Geometry: final body of the model. Coordinates: model frame, mm. Face numbers are marked on the shaded views. A direction names the side the tool comes from. Round coordinates to 2 decimals unless told otherwise and drop trailing zeros. Write each loop counter-clockwise with the first axis right and the second up, starting at its lowest first coordinate (ties: lowest second). Pieces come first, ordered by that corner, then holes. Notation, with made-up numbers: (56, 78.5) -> (72, 78.5) arc R22 ccw to (72, 99.5) -> close; hole circle Ø5 at (-13, 15.5). An arc over 180 degrees is marked (long way). Use one line per item in the form item = value. Start each with the question number.
1. Cut plane B-B, the plane y = 1.25. Return the cut outline in (x, z) (3 decimals), plus the area to 3 significant figures.
2. Line query: L1, parallel to X at y = 3, z = 19; L2, parallel to Z at x = 11.25, y = 4.5; L3, parallel to Y at x = -4, z = -19.05. Output: solid intervals per line, ascending.
3. Cut plane D-D, the plane z = 5. Return the cut outline in (x, y), plus the area to 3 significant figures.
4. Draft query along X for the marked faces 1, 2, 3 and 4. Return one class per face: pulls with the +X half, pulls with the -X half, needs draft (parallel to the pull), parting line crosses it, or undercut.
5. Pin query (flat end, axial travel): pin 1 Ø3 at (x, z) = (8, 4) entering from -Y; pin 2 Ø9.5 at (y, z) = (-13.5, 3.5) entering from +X. Return the tip coordinate at first contact, or that it passes through.
6. Cut plane A-A, the plane z = -19.05. Return the cut outline in (x, y), plus the area to 3 significant figures.
7. Reachability of the marked faces 5 and 6 from +Z, -Z, +X, -X, +Y, -Y: full face, straight path, thin tool, end or side. Return the list, or none.
8. Cut plane C-C, the plane x = 8.75. Return the cut outline in (y, z).
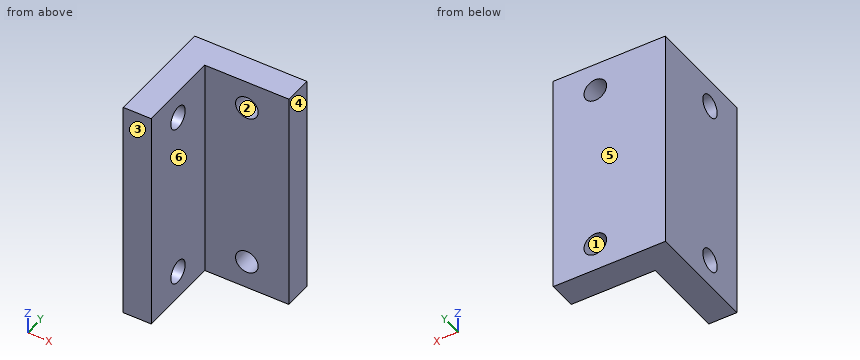
```python
from build123d import *

# Parameters (mm, degrees)
BOSS_EXTRUDE1_DEPTH        = 25.4
F_10_CLEARANCE_HOLE1_D     = 5.1054
F_10_CLEARANCE_HOLE2_D     = 5.1054
F_10_CLEARANCE_HOLE2_DEPTH = 6.35
F_10_CLEARANCE_HOLE2_TIP   = 1.533816902


with BuildPart() as part:
    # Sketch1 → Boss-Extrude1 (new, symmetric)
    with BuildSketch(Plane.XY):
        Polygon((0, 0), (19.05, 0), (19.05, 6.35), (-6.35, 6.35), (-6.35, -19.05), (0, -19.05), align=None)
    extrude(amount=BOSS_EXTRUDE1_DEPTH, both=True)

    # #10 Clearance Hole1 (through all)
    with Locations(Plane(origin=(0, 0, 0), x_dir=(-1, 0, 0), z_dir=(0, -1, 0))):
        with Locations((-9.525, -19.05), (-9.525, 19.05)):
            Hole(F_10_CLEARANCE_HOLE1_D / 2)

    # #10 Clearance Hole2
    with Locations(Plane(origin=(0, 0, 0), x_dir=(0, 0, -1), z_dir=(1, 0, 0))):
        with Locations((19.05, -9.525), (-19.05, -9.525)):
            Hole(F_10_CLEARANCE_HOLE2_D / 2, depth=F_10_CLEARANCE_HOLE2_DEPTH)
            with Locations((0, 0, -(F_10_CLEARANCE_HOLE2_DEPTH + F_10_CLEARANCE_HOLE2_TIP / 2))):  # 118° drill point
                Cone(0, F_10_CLEARANCE_HOLE2_D / 2, F_10_CLEARANCE_HOLE2_TIP, mode=Mode.SUBTRACT)


solid = part.part
```
Outcome:
q1.outline = (-6.35, -25.4) -> (19.05, -25.4) -> (19.05, 25.4) -> (-6.35, 25.4) -> close; hole circle Ø5.105 at (9.525, -19.05); hole circle Ø5.105 at (9.525, 19.05)
q1.area = 1,250 mm^2
q2.L1 = -6.35 to 6.97, 12.08 to 19.05
q2.L2 = -25.4 to -20.93, -17.17 to 17.17, 20.93 to 25.4
q2.L3 = -19.05 to -12.08, -6.97 to 6.35
q3.outline = (-6.35, -19.05) -> (0, -19.05) -> (0, 0) -> (19.05, 0) -> (19.05, 6.35) -> (-6.35, 6.35) -> close
q3.area = 282 mm^2
q4.face_1 = undercut
q4.face_2 = undercut
q4.face_3 = needs draft
q4.face_4 = pulls with the +X half
q5.pin_1 = 0
q5.pin_2 = 0
q6.outline = (-6.35, -19.05) -> (0, -19.05) -> (0, -12.08) -> (-6.35, -12.08) -> close; (-6.35, -6.97) -> (0, -6.97) -> (0, 0) -> (6.97, 0) -> (6.97, 6.35) -> (-6.35, 6.35) -> close; (12.08, 0) -> (19.05, 0) -> (19.05, 6.35) -> (12.08, 6.35) -> close
q6.area = 217 mm^2
q7.face_5 = +Z, -Z, +X, -X, +Y
q7.face_6 = +Z, -Z, +X, -Y
q8.outline = (0, -25.4) -> (6.35, -25.4) -> (6.35, -21.48) -> (0, -21.48) -> close; (0, -16.62) -> (6.35, -16.62) -> (6.35, 16.62) -> (0, 16.62) -> close; (0, 21.48) -> (6.35, 21.48) -> (6.35, 25.4) -> (0, 25.4) -> close
